from build123d import *

# Parameters (mm, degrees)
BOSS_EXTRUDE1_DEPTH     = 125
BOSS_EXTRUDE3_DEPTH     = 1
TAP_DRILL_FOR_M8_TAP1_D = 6.8
SKETCH7_R               = 11.28805381
CUT_EXTRUDE1_DEPTH      = 1
SKETCH8_W               = 17.605373939
SKETCH8_H               = 74.840918302
CUT_EXTRUDE2_DEPTH      = 1


with BuildPart() as part:
    # Sketch1 → Boss-Extrude1 (new body, symmetric)
    with BuildSketch(Plane.XY):
        Polygon((-13.181947142, 17.7), (-13.181947142, 47.7), (61.818052858, 47.7), (61.818052858, -2.3), (79.818052858, -2.3), (79.818052858, -1.3), (62.818052858, -1.3), (62.818052858, 48.7), (-14.181947142, 48.7), (-14.181947142, 17.7), align=None)
    extrude(amount=BOSS_EXTRUDE1_DEPTH, both=True)

    # Sketch2 → Boss-Extrude3 (add)
    with BuildSketch(Plane.XZ.offset(2.3)):
        Polygon((79.818052858, 125), (79.818052858, 50), (140.446405645, 100), (140.446405645, 125), align=None)
        Polygon((79.818052858, -50), (79.818052858, -125), (140.446405645, -125), (140.446405645, -100), align=None)
    extrude(amount=-BOSS_EXTRUDE3_DEPTH)

    # Tap Drill for M8 Tap1 (through all)
    with Locations(Plane(origin=(0, -2.3, 0), x_dir=(-1, 0, 0), z_dir=(0, -1, 0))):
        with Locations((-125.446405645, 110), (-109.974750597, -118.548748507)):
            Hole(TAP_DRILL_FOR_M8_TAP1_D / 2)

    # Sketch7 → Cut-Extrude1 (cut)
    with BuildSketch(Plane.XZ.offset(2.3)):
        with Locations((91.223262411, 73.278651414)):
            Circle(SKETCH7_R)
    extrude(amount=-CUT_EXTRUDE1_DEPTH, mode=Mode.SUBTRACT)

    # Sketch8 → Cut-Extrude2 (cut)
    with BuildSketch(Plane.XZ.offset(2.3)):
        with Locations((79.721629834, -0.077471799)):
            Rectangle(SKETCH8_W, SKETCH8_H)
    extrude(amount=-CUT_EXTRUDE2_DEPTH, mode=Mode.SUBTRACT)


solid = part.part
Here's how the part is built. I have some questions about the finished solid (model axes, mm). A direction names the side the tool comes from. Coordinates: 2 decimals unless noted, no trailing zeros. Write each loop counter-clockwise with the first axis right and the second up, starting at its lowest first coordinate (ties: lowest second). Pieces come first, ordered by that corner, then holes.
1) If we section it at C-C (x = 84.5): List the corners of the cut face in (y, z) for me, plus the area to 3 significant figures.
Filled in:
outline: (-2.3, -125) - (-1.3, -125) - (-1.3, -53.86) - (-2.3, -53.86) - close; (-2.3, 53.86) - (-1.3, 53.86) - (-1.3, 64.21) - (-2.3, 64.21) - close; (-2.3, 82.35) - (-1.3, 82.35) - (-1.3, 125) - (-2.3, 125) - close
area: 124 mm2
2) If we section it at B-B (z = -110): List the corners of the cut face in (x, y) for me.
Filled in:
outline: (-14.18, 17.7) - (-13.18, 17.7) - (-13.18, 47.7) - (61.82, 47.7) - (61.82, -2.3) - (122.05, -2.3) - (122.05, -1.3) - (62.82, -1.3) - (62.82, 48.7) - (-14.18, 48.7) - close; (128.85, -2.3) - (140.45, -2.3) - (140.45, -1.3) - (128.85, -1.3) - close
3) If I drill on line 1 (X direction, y = 26, z = -2); line 2 (Y direction, x = -7, z = 42.5); line 3 (X direction, y = 14.5, z = 26), over which ranges is the centre line in solid material (lowest first)?
Filled in:
line 1: x = -14.18 to -13.18, 61.82 to 62.82
line 2: y = 47.7 to 48.7
line 3: x = 61.82 to 62.82
4) Which directions (+Z, -Z, +X, -X, +Y, -Y) give clear straight access to the entire face, cutting with the end or side of a thin tool? Please do faces 1 (the face through (62.818, 23, 2)), 2 (the face through (110.557, -1.807, -75.35)), 3 (the face through (24, 47.7, 2)).
Filled in:
face 1: +Z, -Z, +X, +Y
face 2: +X, +Y, -Y
face 3: +Z, -Z, -Y
5) If we section it at A-A (y = 25.5): List the corners of the cut face in (x, z) for me, plus the area to 3 significant figures.
Filled in:
outline: (-14.18, -125) - (-13.18, -125) - (-13.18, 125) - (-14.18, 125) - close; (61.82, -125) - (62.82, -125) - (62.82, 125) - (61.82, 125) - close
area: 500 mm2
6) If we section it at D-D (z = 24): List the corners of the cut face in (x, y) for me.
Filled in:
outline: (-14.18, 17.7) - (-13.18, 17.7) - (-13.18, 47.7) - (61.82, 47.7) - (61.82, -2.3) - (70.92, -2.3) - (70.92, -1.3) - (62.82, -1.3) - (62.82, 48.7) - (-14.18, 48.7) - close
7) Thinking about a two-plate mould opening in Z: for faces 4 (the face through (67, -1.3, 2)), 5 (the face through (103.6, -1.5, 125)), 6 (the face through (120.346, -1.807, 83.423)), which applies, +Z half, -Z half, draft (parallel to the pull), parting line (faces both ways), or undercut?
Filled in:
face 4: draft
face 5: +Z half
face 6: undercut
8) I'm going to push flat-ended pins straight in: pin 1 (9 mm diameter, centred on x = 109.97, z = 118.55, fed in from -Y); pin 2 (1.1 mm diameter, centred on y = -2, z = 43.5, fed in from +X); pin 3 (10 mm diameter, centred on x = 39.5, z = 97.5, fed in from -Y); pin 4 (1.1 mm diameter, centred on y = -2, z = 1, fed in from +X). Where does each tip first touch, or does it pass through?
Filled in:
pin 1: stops at y = -2.3
pin 2: stops at x = 79.82
pin 3: stops at y = 47.7
pin 4: stops at x = 70.92
